```python
from build123d import *

# Parameters (mm, degrees)
SKETCH1_W               = 289.56
SKETCH1_H               = 289.56
BOSS_EXTRUDE1_DEPTH     = 12.7
SKETCH7_R               = 127.635
SKETCH7_R_2             = 123.19
CUT_EXTRUDE1_DEPTH      = 9.525
F_1_4_CLEARANCE_HOLE1_D = 6.7564
CIRPATTERN1_COUNT       = 4


with BuildPart() as part:
    # Sketch1 → Boss-Extrude1 (new body)
    with BuildSketch(Plane(origin=(0, 0, 0), x_dir=(1, 0, 0), z_dir=(0, 1, 0))):
        Rectangle(SKETCH1_W, SKETCH1_H)
    extrude(amount=BOSS_EXTRUDE1_DEPTH)

    # Sketch7 → Cut-Extrude1 (cut)
    with BuildSketch(Plane(origin=(0, 12.7, 0), x_dir=(1, 0, 0), z_dir=(0, 1, 0))):
        Circle(SKETCH7_R)
        Circle(SKETCH7_R_2, mode=Mode.SUBTRACT)
    extrude(amount=-CUT_EXTRUDE1_DEPTH, mode=Mode.SUBTRACT)

    # 1/4 Clearance Hole1 (through all)
    with Locations(Plane(origin=(0, 0, 0), x_dir=(-1, 0, 0), z_dir=(0, -1, 0))):
        with Locations((98.782817332, -98.782817332)):
            f_1_4_clearance_hole1 = Hole(F_1_4_CLEARANCE_HOLE1_D / 2)

    # CirPattern1: 1/4 Clearance Hole1 ×4 about axis
    cirpattern1_axis = Axis((0, 0, 0), (0, 1, 0))
    for i in range(1, CIRPATTERN1_COUNT):
        add(f_1_4_clearance_hole1.rotate(cirpattern1_axis, i * 360 / CIRPATTERN1_COUNT), mode=Mode.SUBTRACT)


solid = part.part
```
Part model, mm, in its own coordinate system. A direction names the side the tool comes from. Round coordinates to 2 decimals unless told otherwise and drop trailing zeros. Loops run counter-clockwise (first coordinate to the right, second up) from the corner with the lowest first, then second, coordinate; pieces in that order, holes last. Notation, with made-up numbers: (82, 11) -> (99, 11) arc R23 cw to (99, 23) -> close; hole circle Ø1 at (35, -29.5). An arc over 180 degrees is marked (long way). Use CSV: the item, a comma, the result in double quotes. Start each with the question number.
1) Which spindle directions (+Z, -Z, +X, -X, +Y, -Y) get a long thin tool onto all of the face, cutting with end or side? Do faces 4 (the flat face through (-67, 3.175, -105)), 5 (the flat face through (-131, 12.7, -2)). Say none if no direction does.
2) Wall check: L1, parallel to Z at x = -3, y = 7.25; L2, parallel to X at y = 6.25, z = 0 (3 decimals); L3, parallel to Z at x = -88.5, y = 6.5. Give the ranges that are in metal, low to high. Write a range as [from, to].
3) Cut at B-B, the plane x = 0. Write the cut outline in (y, z) (3 decimals).
4) Cut at C-C, the plane z = 0. Write the cut outline in (x, y) (3 decimals), plus the area to 3 significant figures.
5) Drop a flat-ended pin along its axis: P1, Ø5.5, axis at x = 98.78, z = -98.78, coming from the -Y side. Give the stop position or say it passes through.
6) Pull direction X, two halves, no side cores. Call faces 1 (the cylindrical face through (-101.273, 6.439, 96.5)), 2 (the flat face through (-2, 0, -2)), 3 (the flat face through (144.78, 6, 2)): +X half, -X half, draft (parallel to the pull), parting line (faces both ways), or undercut.
7) Cut at A-A, the plane y = 5.25. Write the cut outline in (x, z) (3 decimals), plus the area to 3 significant figures.
Determined:
1,face 4,"+Y"
1,face 5,"+Z, -Z, +X, -X, +Y"
2,L1,"z = [-144.78, -127.6], [-123.15, 123.15], [127.6, 144.78]"
2,L2,"x = [-144.78, -127.635], [-123.19, 123.19], [127.635, 144.78]"
2,L3,"z = [-144.78, -91.97], [-85.69, 85.69], [91.97, 144.78]"
3,outline,"(0, -144.78) -> (12.7, -144.78) -> (12.7, -127.635) -> (3.175, -127.635) -> (3.175, -123.19) -> (12.7, -123.19) -> (12.7, 123.19) -> (3.175, 123.19) -> (3.175, 127.635) -> (12.7, 127.635) -> (12.7, 144.78) -> (0, 144.78) -> close"
4,outline,"(-144.78, 0) -> (144.78, 0) -> (144.78, 12.7) -> (127.635, 12.7) -> (127.635, 3.175) -> (123.19, 3.175) -> (123.19, 12.7) -> (-123.19, 12.7) -> (-123.19, 3.175) -> (-127.635, 3.175) -> (-127.635, 12.7) -> (-144.78, 12.7) -> close"
4,area,"3,590 mm2"
5,P1,"passes through"
6,face 1,"undercut"
6,face 2,"draft"
6,face 3,"+X half"
7,outline,"(-144.78, -144.78) -> (144.78, -144.78) -> (144.78, 144.78) -> (-144.78, 144.78) -> close; circle Ø246.38 at (0, 0); hole circle Ø255.27 at (0, 0); hole circle Ø6.756 at (-98.783, -98.783); hole circle Ø6.756 at (-98.783, 98.783); hole circle Ø6.756 at (98.783, -98.783); hole circle Ø6.756 at (98.783, 98.783)"
7,area,"80,200 mm2"
